Check sheet for the modelled part. Datum: model origin and axes. Units: mm. Face numbers are marked on the shaded views. A direction names the side the tool comes from. Coordinates: 2 decimals unless noted, no trailing zeros. Write each loop counter-clockwise with the first axis right and the second up, starting at its lowest first coordinate (ties: lowest second). Pieces come first, ordered by that corner, then holes. Notation, with made-up numbers: (-40, 30.5) -> (-14, 30.5) arc R17 ccw to (-14, 44.5) -> close; hole circle Ø4 at (-2.75, 46). An arc over 180 degrees is marked (long way). One line per item, written item: value. Start each with the question number.
1) Set-up check for the marked faces 4, 5 and 6: record each of +Z, -Z, +X, -X, +Y, -Y from which the full face is reachable in a straight line by a thin tool's end or side.
2) Sectioned sample at A-A on x = -25.5. Enter the section's corners in (y, z), plus the area to 3 significant figures.
3) Sectioned sample at B-B on y = -2.5. Enter the section's corners in (x, z), plus the area to 3 significant figures.
4) Draft check along X on the marked faces 1, 2 and 3. Enter one of: +X half, -X half, draft (parallel to the pull), parting line (faces both ways), or undercut.
5) Sectioned sample at D-D on x = -3. Enter the section's corners in (y, z), plus the area to 3 significant figures.
6) Scan lines: line 1 along X through (y, z) = (1.25, 5); line 2 along X through (y, z) = (1.75, 5); line 3 along Y through (x, z) = (-11, 8.5). Record each from-to range of solid material in increasing order. Write a range as [from, to].
7) Gauge pin test, flat ends, axial feed: P1, Ø3, axis at x = -38, z = 3.5, coming from the -Y side; P2, Ø0.9, axis at y = -13.5, z = 2, coming from the -X side; P3, Ø5, axis at y = -11.5, z = 1, coming from the -X side. Record the tip position at first contact, or that the pin passes through.
8) Sectioned sample at C-C on z = 9.25. Enter the section's corners in (x, y), plus the area to 3 significant figures.
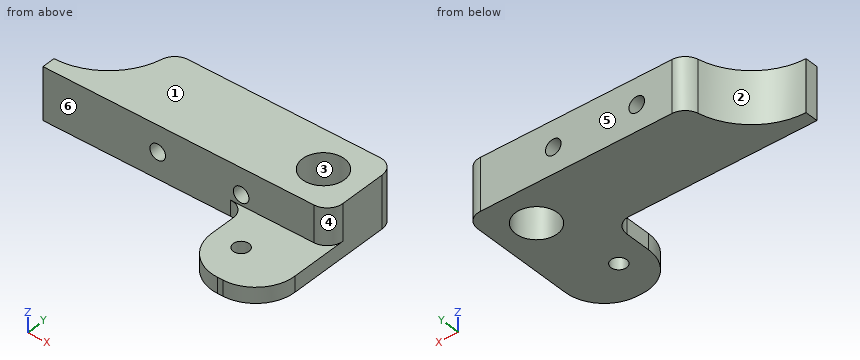
```python
from build123d import *

# Parameters (mm, degrees)
CROQUIS1_R              = 4
SALIENTE_EXTRUIR1_DEPTH = 10
CROQUIS3_W              = 16
CROQUIS3_H              = 15.5
CROQUIS3_R              = 1.5
SALIENTE_EXTRUIR2_DEPTH = 3
REDONDEO1_R             = 7.5
REDONDEO2_R             = 3
CROQUIS4_R              = 1.5
CORTAR_EXTRUIR2_DEPTH   = 15
REDONDEO3_R             = 3


with BuildPart() as part:
    # Croquis1 → Saliente-Extruir1 (new body)
    with BuildSketch(Plane.XY):
        with BuildLine():
            Line((-35, 7.5), (7.5, 7.5))
            Line((7.5, 7.5), (7.5, -7.5))
            Line((7.5, -7.5), (-47.5, -7.5))
            Line((-47.5, -7.5), (-47.5, -5))
            ThreePointArc((-47.5, -5), (-38.661165235, -1.338834765), (-35, 7.5))
        make_face()
        Circle(CROQUIS1_R, mode=Mode.SUBTRACT)
    extrude(amount=SALIENTE_EXTRUIR1_DEPTH)

    # Croquis3 → Saliente-Extruir2 (add)
    with BuildSketch(Plane.XY):
        with Locations((-0.5, -15.25)):
            Rectangle(CROQUIS3_W, CROQUIS3_H)
        with Locations((-3, -15.25)):
            Circle(CROQUIS3_R, mode=Mode.SUBTRACT)
    extrude(amount=SALIENTE_EXTRUIR2_DEPTH)

    # Redondeo1
    redondeo1_edges = [part.edges().sort_by_distance(p)[0] for p in [
        (7.5, -23, 1.5),
        (-8.5, -23, 1.5),
    ]]
    fillet(redondeo1_edges, radius=REDONDEO1_R)

    # Redondeo2
    redondeo2_edges = [part.edges().sort_by_distance(p)[0] for p in [
        (-8.5, -7.5, 1.5),
    ]]
    fillet(redondeo2_edges, radius=REDONDEO2_R)

    # Croquis4 → Cortar-Extruir2 (cut)
    with BuildSketch(Plane(origin=(0, 7.5, 0), x_dir=(1, 0, 0), z_dir=(0, 1, 0))):
        with Locations(Location((-25.5, -5, 0), (0, 0, 270))):
            Circle(CROQUIS4_R)
        with Locations(Location((-9.5, -5, 0), (0, 0, 270))):
            Circle(CROQUIS4_R)
    extrude(amount=-CORTAR_EXTRUIR2_DEPTH, mode=Mode.SUBTRACT)

    # Redondeo3
    redondeo3_edges = [part.edges().sort_by_distance(p)[0] for p in [
        (7.5, -7.5, 6.5),
        (-35, 7.5, 5),
        (7.5, 7.5, 5),
    ]]
    fillet(redondeo3_edges, radius=REDONDEO3_R)


solid = part.part
```
Answers:
1. face 4: +Z, +X, -Y
1. face 5: +Z, -Z, +X, -X, +Y
1. face 6: +Z, -X, -Y
2. outline: (-7.5, 0) -> (7.5, 0) -> (7.5, 3.5) -> (-7.5, 3.5) -> close; (-7.5, 6.5) -> (7.5, 6.5) -> (7.5, 10) -> (-7.5, 10) -> close
2. area: 105 mm2
3. outline: (-40, 0) -> (-3.12, 0) -> (-3.12, 10) -> (-40, 10) -> close; (3.12, 0) -> (7.5, 0) -> (7.5, 10) -> (3.12, 10) -> close; hole circle Ø3 at (-25.5, 5); hole circle Ø3 at (-9.5, 5)
3. area: 398 mm2
4. face 1: draft
4. face 2: -X half
4. face 3: undercut
5. outline: (-22.73, 0) -> (-16.75, 0) -> (-16.75, 3) -> (-22.73, 3) -> close; (-13.75, 0) -> (-2.65, 0) -> (-2.65, 10) -> (-7.5, 10) -> (-7.5, 3) -> (-13.75, 3) -> close; (2.65, 0) -> (7.5, 0) -> (7.5, 10) -> (2.65, 10) -> close
5. area: 134 mm2
6. line 1: x = [-36.67, -27], [-24, -11], [-8, -3.8], [3.8, 7.5]
6. line 2: x = [-36.4, -27], [-24, -11], [-8, -3.6], [3.6, 7.5]
6. line 3: y = [-7.5, 7.5]
7. P1: stops at y = -7.5
7. P2: stops at x = -8.5
7. P3: stops at x = -8.9
8. outline: (-47.5, -7.5) -> (4.5, -7.5) arc R3 ccw to (7.5, -4.5) -> (7.5, 4.5) arc R3 ccw to (4.5, 7.5) -> (-32.29, 7.5) arc R3 ccw to (-35.24, 5.08) arc R12.5 cw to (-47.5, -5) -> close; hole circle Ø8 at (0, 0)
8. area: 647 mm2
